```python
from build123d import *

# Parameters (mm, degrees)
SKETCH1_W                    = 38.1
SKETCH1_H                    = 38.1
SKETCH1_W_2                  = 31.75
SKETCH1_H_2                  = 31.75
BOSS_EXTRUDE1_DEPTH          = 95.25
F_10_0_1935_DIAMETER_HOLE1_D = 4.9149


with BuildPart() as part:
    # Sketch1 → Boss-Extrude1 (new body)
    with BuildSketch(Plane.XY):
        Rectangle(SKETCH1_W, SKETCH1_H)
        Rectangle(SKETCH1_W_2, SKETCH1_H_2, mode=Mode.SUBTRACT)
    extrude(amount=BOSS_EXTRUDE1_DEPTH)

    # #10 (0.1935) Diameter Hole1 (through all)
    with Locations(Plane(origin=(19.05, 0, 19.05), x_dir=(0, 0, 1), z_dir=(1, 0, 0))):
        with Locations((0, 0), (57.15, 0), (28.575, 0)):
            Hole(F_10_0_1935_DIAMETER_HOLE1_D / 2)


solid = part.part
```
Geometry: final body of the model. Coordinates: model frame, mm. A direction names the side the tool comes from. Round coordinates to 2 decimals unless told otherwise and drop trailing zeros. Write each loop counter-clockwise with the first axis right and the second up, starting at its lowest first coordinate (ties: lowest second). Pieces come first, ordered by that corner, then holes. Notation, with made-up numbers: (88.25, 65) -> (104.25, 65) arc R12 cw to (104.25, 76) -> close; hole circle Ø6 at (4, -11). An arc over 180 degrees is marked (long way). Return JSON: item names as keys, results as strings.
Q1. First-contact query: pin 1 Ø3 at (y, z) = (0, 76.2) entering from -X. Flat tip, straight axial feed; report the tip coordinate or a pass-through.
From the geometry:
{"pin 1": "through"}
Q2. Ray query, line 1 (X direction, y = 10, z = 67.5) (3 decimals); line 2 (Y direction, x = -17, z = 19). Return the intervals inside material, ascending.
From the geometry:
{"line 1": "-19.05 to -15.875, 15.875 to 19.05", "line 2": "-19.05 to -2.46, 2.46 to 19.05"}
Q3. Section B-B on x = 7. Return the cut outline in (y, z) (3 decimals), and give its area (3 significant figures).
From the geometry:
{"outline": "(-19.05, 0) -> (-15.875, 0) -> (-15.875, 95.25) -> (-19.05, 95.25) -> close; (15.875, 0) -> (19.05, 0) -> (19.05, 95.25) -> (15.875, 95.25) -> close", "area": "605 mm2"}
Q4. Set-up query: faces 5 (the cylindrical face through (-17.485, 1.495, 49.575)), 6 (the flat face through (0, -15.875, 47)). Return all of +Z, -Z, +X, -X, +Y, -Y with unobstructed straight access to the full face (end or side cutting, diameter ignored); none if empty.
From the geometry:
{"face 5": "+X, -X", "face 6": "+Z, -Z"}
Q5. Section A-A on z = 19.05. Return the cut outline in (x, y) (3 decimals), and give its area (3 significant figures).
From the geometry:
{"outline": "(-19.05, -19.05) -> (19.05, -19.05) -> (19.05, -2.457) -> (15.875, -2.457) -> (15.875, -15.875) -> (-15.875, -15.875) -> (-15.875, -2.457) -> (-19.05, -2.457) -> close; (-19.05, 2.457) -> (-15.875, 2.457) -> (-15.875, 15.875) -> (15.875, 15.875) -> (15.875, 2.457) -> (19.05, 2.457) -> (19.05, 19.05) -> (-19.05, 19.05) -> close", "area": "412 mm2"}
Q6. Mould query, pull axis X, two halves, no side actions, for faces 1 (the flat face through (19.05, 4, 47)), 2 (the flat face through (0, 15.875, 47)), 3 (the cylindrical face through (17.44, -0.738, 16.706)), 4 (the flat face through (15.875, 3, 47)). Classes: +X half, -X half, draft (parallel to the pull), parting line (faces both ways), or undercut.
From the geometry:
{"face 1": "+X half", "face 2": "undercut", "face 3": "draft", "face 4": "undercut"}
Q7. Section C-C on y = 0. Give the number of separate pieces and of enclosed holes in the cut face, and give its area (3 significant figures).
From the geometry:
{"separate pieces": "8", "enclosed holes": "0", "area": "511 mm2"}
